from build123d import *

# Parameters (mm, degrees)
SKETCH1_W           = 254
SKETCH1_H           = 203.2
BOSS_EXTRUDE1_DEPTH = 6.35
SKETCH2_R           = 14.2748
SKETCH2_W           = 25.4
SKETCH2_H           = 101.6
CUT_EXTRUDE1_DEPTH  = 163.763271348


with BuildPart() as part:
    # Sketch1 → Boss-Extrude1 (new body)
    with BuildSketch(Plane.XY):
        Rectangle(SKETCH1_W, SKETCH1_H)
    extrude(amount=BOSS_EXTRUDE1_DEPTH)

    # Sketch2 → Cut-Extrude1 (cut, through all)
    with BuildSketch(Plane.XY.offset(6.35)):
        with Locations((71.12, 74.93)):
            Circle(SKETCH2_R)
        with Locations((-114.3, -50.8)):
            Rectangle(SKETCH2_W, SKETCH2_H)
    extrude(amount=-CUT_EXTRUDE1_DEPTH, mode=Mode.SUBTRACT)


solid = part.part
Source: CAD feature listing. Evaluate the final solid. Frame: model axes, mm. A direction names the side the tool comes from. Round coordinates to 2 decimals unless told otherwise and drop trailing zeros. Loops run counter-clockwise (first coordinate to the right, second up) from the corner with the lowest first, then second, coordinate; pieces in that order, holes last. Notation, with made-up numbers: (51.25, -26) - (70.25, -26) arc R11 ccw to (70.25, -22) - close; hole circle Ø11 at (38, -6.5). An arc over 180 degrees is marked (long way). Write item = value, one per line. Start each with the question number.
Item 1: First-contact query: pin 1 Ø1.9 at (x, z) = (-109.5, 2.5) entering from -Y; pin 2 Ø1.9 at (y, z) = (-38, 2.5) entering from -X. Flat tips, straight axial feed; report the tip coordinate or a pass-through.
Item 2: Reachability of faces 1 (the face through (-101.6, -52, 3)), 2 (the face through (127, -1, 3)) from +Z, -Z, +X, -X, +Y, -Y: full face, straight path, thin tool, end or side. Return the list, or none.
Item 3: Section query D-D on y = -21. Output: boundary loops of the cut face in (x, z), plus the area to 3 significant figures.
Item 4: Section query C-C on z = 1. Output: boundary loops of the cut face in (x, y), plus the area to 3 significant figures.
Item 5: Mould query, pull axis Y, two halves, no side actions, for faces 3 (the face through (59.792, 66.244, 3.219)), 4 (the face through (-2, 1, 0)), 5 (the face through (11, -101.6, 3)). Classes: released by +Y, released by -Y, zero draft, split by the parting line, or undercut.
Item 6: Material intervals for line 1 (X direction, y = -9.5, z = 4); line 2 (Y direction, x = -103.5, z = 4); line 3 (Y direction, x = 71.12, z = 2.25), sorted ascending.
Item 7: Section query A-A on x = 71.12. Output: boundary loops of the cut face in (y, z), plus the area to 3 significant figures.
Item 8: Section query B-B on y = 74.93. Output: boundary loops of the cut face in (x, z).
Results list:
q1.pin_1 = 0
q1.pin_2 = -101.6
q2.face_1 = +Z, -Z, -X, -Y
q2.face_2 = +Z, -Z, +X, +Y, -Y
q3.outline = (-101.6, 0) - (127, 0) - (127, 6.35) - (-101.6, 6.35) - close
q3.area = 1,450 mm²
q4.outline = (-127, 0) - (-101.6, 0) - (-101.6, -101.6) - (127, -101.6) - (127, 101.6) - (-127, 101.6) - close; hole circle Ø28.55 at (71.12, 74.93)
q4.area = 48,400 mm²
q5.face_3 = undercut
q5.face_4 = zero draft
q5.face_5 = released by -Y
q6.line_1 = -101.6 to 127
q6.line_2 = 0 to 101.6
q6.line_3 = -101.6 to 60.66, 89.2 to 101.6
q7.outline = (-101.6, 0) - (60.66, 0) - (60.66, 6.35) - (-101.6, 6.35) - close; (89.2, 0) - (101.6, 0) - (101.6, 6.35) - (89.2, 6.35) - close
q7.area = 1,110 mm²
q8.outline = (-127, 0) - (56.85, 0) - (56.85, 6.35) - (-127, 6.35) - close; (85.39, 0) - (127, 0) - (127, 6.35) - (85.39, 6.35) - close
